Verification items for this drawing (mm, ordinates from the low corner). Coordinates: 2 decimals unless noted, no trailing zeros. Write item = value, one per line.
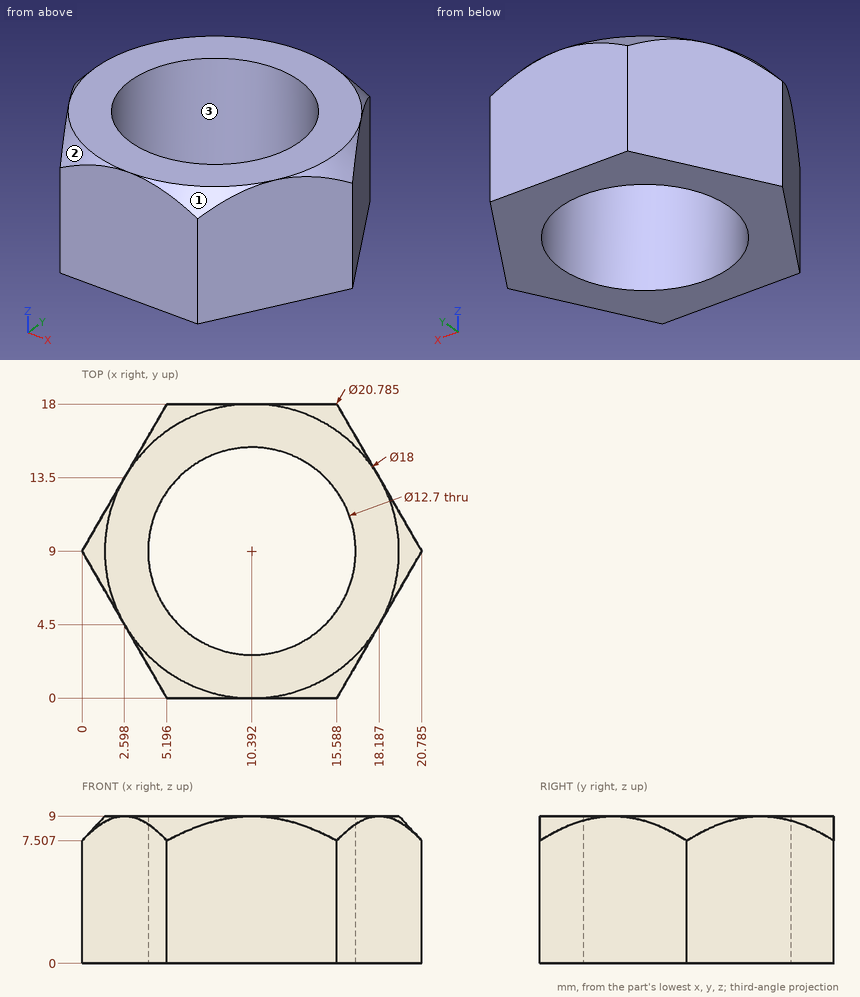
Item 1: Gauge pin test, flat ends, axial feed: pin 1 (3 mm diameter, centred on y = 13.5, z = 3, fed in from +X); pin 2 (1 mm diameter, centred on y = 8, z = 2, fed in from +X) (1 decimal). Record the tip position at first contact, or that the pin passes through.
Report:
pin_1 = 19.05
pin_2 = 20.5
Item 2: Scan lines: L1, parallel to X at y = 10, z = 6.75 (1 decimal); L2, parallel to X at y = 11.25, z = 2 (1 decimal); L3, parallel to Y at x = 12, z = 1.75. Record each from-to range of solid material in increasing order. Write a range as from..to.
Report:
L1 = 0.6..4.1, 16.7..20.2
L2 = 1.3..4.5, 16.3..19.5
L3 = 0..2.86, 15.14..18
Item 3: Release check for a two-part mould opening along X. For the marked faces 1, 2 and 3 record: pulls with the +X half, pulls with the -X half, needs draft (parallel to the pull), parting line crosses it, or undercut.
Report:
face_1 = pulls with the +X half
face_2 = pulls with the -X half
face_3 = undercut
